Could you check a few things on this model? Use its own coordinates, in mm. A direction names the side the tool comes from. Coordinates: 2 decimals unless noted, no trailing zeros. Order: outer loops, then holes, each group sorted by start corner. A loop starts at its lowest first (then second) coordinate and runs counter-clockwise, first axis right, second up. Notation, with made-up numbers: (53.25, 39.5) -> (108.25, 39.5) arc R14 cw to (108.25, 65.5) -> close; hole circle Ø2 at (-27, 69.5). An arc over 180 degrees is marked (long way). Use a Markdown table: item, result. Add a question column.
1) If I drill on L1, parallel to Z at x = 11, y = 3.5; L2, parallel to Z at x = 39, y = 2.8, over which ranges is the centre line in solid material (lowest first)? Write a range as [from, to].
2) Which directions (+Z, -Z, +X, -X, +Y, -Y) give clear straight access to the entire face, cutting with the end or side of a thin tool? Please do faces 1 (the flat face through (22, 2, 0)), 2 (the flat face through (7, 2, 22.1)).
3) If we section it at C-C (y = 3.3): Write out the boundary of the cut face in (x, z).
4) If we section it at A-A (x = 13): Write out the boundary of the cut face in (y, z), plus the area to 3 significant figures.
5) If we section it at B-B (z = 38): Write out the boundary of the cut face in (x, y), plus the area to 3 significant figures.
6) Thinking about a two-plate mould opening in Z: for faces 3 (the flat face through (22, 2, 45)), 4 (the flat face through (17, 0, 7)), 5 (the flat face through (22.9, 2, 38)), which applies, +Z half, -Z half, draft (parallel to the pull), parting line (faces both ways), or undercut?
```python
from build123d import *

# Parameters (mm, degrees)
CROQUIS1_W              = 45
CROQUIS1_H              = 45
CROQUIS1_W_2            = 28
CROQUIS1_H_2            = 28
SALIENTE_EXTRUIR1_DEPTH = 5
CROQUIS2_W              = 0.8
CROQUIS2_H              = 3
CROQUIS2_W_2            = 3
CROQUIS2_H_2            = 0.8
CORTAR_EXTRUIR1_DEPTH   = 5


with BuildPart() as part:
    # Croquis1 → Saliente-Extruir1 (new body)
    with BuildSketch(Plane(origin=(0, 0, 0), x_dir=(1, 0, 0), z_dir=(0, 1, 0))):
        with Locations((22.5, -22.5)):
            Rectangle(CROQUIS1_W, CROQUIS1_H)
        with Locations((22.5, -22.5)):
            Rectangle(CROQUIS1_W_2, CROQUIS1_H_2, mode=Mode.SUBTRACT)
    extrude(amount=SALIENTE_EXTRUIR1_DEPTH)

    # Croquis2 → Cortar-Extruir1 (cut)
    with BuildSketch(Plane.XZ):
        with Locations((22.5, 38)):
            Rectangle(CROQUIS2_W, CROQUIS2_H)
        with Locations((38, 22.5)):
            Rectangle(CROQUIS2_W_2, CROQUIS2_H_2)
        with Locations((22.5, 7)):
            Rectangle(CROQUIS2_W, CROQUIS2_H)
        with Locations((7, 22.5)):
            Rectangle(CROQUIS2_W_2, CROQUIS2_H_2)
    extrude(amount=-CORTAR_EXTRUIR1_DEPTH, mode=Mode.SUBTRACT)


solid = part.part
```
Answer sheet:
| question | item | result |
|---|---|---|
| 1 | L1 | [0, 8.5], [36.5, 45] |
| 1 | L2 | [0, 22.1], [22.9, 45] |
| 2 | face 1 | -Z, +X, -X, +Y, -Y |
| 2 | face 2 | +Y, -Y |
| 3 | outline | (0, 0) -> (45, 0) -> (45, 45) -> (0, 45) -> close; hole (5.5, 22.1) -> (8.5, 22.1) -> (8.5, 8.5) -> (22.1, 8.5) -> (22.1, 5.5) -> (22.9, 5.5) -> (22.9, 8.5) -> (36.5, 8.5) -> (36.5, 22.1) -> (39.5, 22.1) -> (39.5, 22.9) -> (36.5, 22.9) -> (36.5, 36.5) -> (22.9, 36.5) -> (22.9, 39.5) -> (22.1, 39.5) -> (22.1, 36.5) -> (8.5, 36.5) -> (8.5, 22.9) -> (5.5, 22.9) -> close |
| 4 | outline | (0, 0) -> (5, 0) -> (5, 8.5) -> (0, 8.5) -> close; (0, 36.5) -> (5, 36.5) -> (5, 45) -> (0, 45) -> close |
| 4 | area | 85.0 mm2 |
| 5 | outline | (0, 0) -> (22.1, 0) -> (22.1, 5) -> (0, 5) -> close; (22.9, 0) -> (45, 0) -> (45, 5) -> (22.9, 5) -> close |
| 5 | area | 221 mm2 |
| 6 | face 3 | +Z half |
| 6 | face 4 | draft |
| 6 | face 5 | undercut |
